```python
from build123d import *

# Parameters (mm, degrees)
SKETCH1_W           = 25
SKETCH1_H           = 25
BOSS_EXTRUDE1_DEPTH = 8
SKETCH2_R           = 5
BOSS_EXTRUDE2_DEPTH = 132
CHAMFER1_SIZE       = 1


with BuildPart() as part:
    # Sketch1 → Boss-Extrude1 (new body)
    with BuildSketch(Plane(origin=(0, 0, 0), x_dir=(1, 0, 0), z_dir=(0, 1, 0))):
        Rectangle(SKETCH1_W, SKETCH1_H)
    extrude(amount=BOSS_EXTRUDE1_DEPTH)

    # Sketch2 → Boss-Extrude2 (add)
    with BuildSketch(Plane(origin=(0, 8, 0), x_dir=(1, 0, 0), z_dir=(0, 1, 0))):
        with Locations(Location((0, 0, 0), (0, 0, 270))):
            Circle(SKETCH2_R)
    extrude(amount=BOSS_EXTRUDE2_DEPTH)

    # Chamfer1
    chamfer1_edges = [part.edges().sort_by_distance(p)[0] for p in [
        (0, 140, -5),
    ]]
    chamfer(chamfer1_edges, length=CHAMFER1_SIZE)


solid = part.part
```
CAD build for the part. Positions are in the model's coordinates, mm. A direction names the side the tool comes from. Coordinates: 2 decimals unless noted, no trailing zeros. Loops run counter-clockwise (first coordinate to the right, second up) from the corner with the lowest first, then second, coordinate; pieces in that order, holes last. Notation, with made-up numbers: (89, 52) - (107, 52) arc R33 cw to (107, 87) - close; hole circle Ø11 at (62, 72). An arc over 180 degrees is marked (long way). Return JSON: item names as keys, results as strings.
1. Band-saw the part on A-A (x = 0). Give the cut face in (y, z).
Result:
{"outline": "(0, -12.5) - (8, -12.5) - (8, -5) - (139, -5) - (140, -4) - (140, 4) - (139, 5) - (8, 5) - (8, 12.5) - (0, 12.5) - close"}
2. Band-saw the part on D-D (z = -10). Give the cut face in (x, y), and give its area (3 significant figures).
Result:
{"outline": "(-12.5, 0) - (12.5, 0) - (12.5, 8) - (-12.5, 8) - close", "area": "200 mm2"}
3. 3-axis set-ups, long thin cutter, end or side, ignore diameter. For faces 1 (the cylindrical face through (-4.88, 72.58, -1.08)), 2 (the flat face through (0, 4, -12.5)): which of +Z, -Z, +X, -X, +Y, -Y reach the whole face in a straight line?
Result:
{"face 1": "+Y", "face 2": "-Z, +X, -X, +Y, -Y"}
4. Band-saw the part on C-C (y = 105.5). Give the cut face in (x, z).
Result:
{"outline": "circle Ø10 at (0, 0)"}
5. Probe L1, parallel to Y at x = -1.75, z = 4.75; L2, parallel to Z at x = 4, y = 68; L3, parallel to X at y = 89, z = -3.5. List the from-to ranges inside material, lowest first. Write a range as from..to.
Result:
{"L1": "y = 0..8", "L2": "z = -3..3", "L3": "x = -3.57..3.57"}
6. Drop flat-ended pins along their axis: pin 1 (12 mm diameter, centred on x = 4, y = 72.5, fed in from -Z); pin 2 (12 mm diameter, centred on x = -2, y = 86.5, fed in from +Z); pin 3 (3 mm diameter, centred on x = 0.5, z = -9.5, fed in from +Y). Give the stop position or say it passes through.
Result:
{"pin 1": "stops at z = -5", "pin 2": "stops at z = 5", "pin 3": "stops at y = 8"}
7. Band-saw the part on B-B (z = 0). Give the cut face in (x, y).
Result:
{"outline": "(-12.5, 0) - (12.5, 0) - (12.5, 8) - (5, 8) - (5, 139) - (4, 140) - (-4, 140) - (-5, 139) - (-5, 8) - (-12.5, 8) - close"}
